Could you check a few things on this model? Use its own coordinates, in mm. Face numbers are marked on the shaded views. Give positions to 0.01 mm unless a question says otherwise; leave off trailing zeros. Loops run counter-clockwise (first coordinate to the right, second up) from the corner with the lowest first, then second, coordinate; pieces in that order, holes last. Notation, with made-up numbers: (-10.75, 80.25) - (42.25, 80.25) arc R30 cw to (42.25, 113.25) - close; hole circle Ø9 at (-9, -6.75). An arc over 180 degrees is marked (long way). Write each question's results on one line, items separated by ' | '. Start each with the question number.
(1) I need wall thicknesses on line 1 (Y direction, x = -1, z = 2.6); line 2 (X direction, y = 4.5, z = 2.7); line 3 (X direction, y = -0.5, z = 0.8) (3 decimals). Which ranges of each line are inside material? Lowest first, please.
(2) Suppose I cut it at A-A (y = 5.5). Please give me the cut outline in (x, z), and give its area (3 significant figures).
(3) Suppose I cut it at B-B (y = 1.5). Please give me the cut outline in (x, z), and give its area (3 significant figures).
(4) For pin 1 (4 mm diameter, centred on x = 0, y = 0, fed in from +Z); pin 2 (1.5 mm diameter, centred on x = -6.5, z = 1.5, fed in from +Y), each with a flat end and sliding along its axis, tell me the tip position at first contact or that it passes through.
(5) Suppose I cut it at C-C (x = 0). Please give me the cut outline in (y, z).
(6) Suppose I cut it at D-D (y = -7.5). Please give me the cut outline in (x, z), and give its area (3 significant figures).
(7) If we mould it in two halves opening along Y, with no side actions, what happens to the marked faces 1, 2, 3 and 4? For each: released by +Y, released by -Y, zero draft, split by the parting line, or undercut.
from build123d import *

# Parameters (mm, degrees)
SKETCH_1_R      = 3
SKETCH_1_R_2    = 0.8
SKETCH_1_R_3    = 1.25
EXTRUDE_1_DEPTH = 3
FILLET_1_R      = 0.5
FILLET_2_R      = 1


with BuildPart() as part:
    # ｽｹｯﾁ1 → ﾎﾞｽ - 押し出し1 (new body)
    with BuildSketch(Plane.XY):
        with BuildLine():
            ThreePointArc((-11.50012809, -9.630527187), (-15.242047107, -8.8), (-14.090345241, -5.144139479))
            ThreePointArc((-14.090345241, -5.144139479), (-12.990381057, 7.5), (-2.590217151, 14.774666667))
            ThreePointArc((-2.590217151, 14.774666667), (0, 17.6), (2.590217151, 14.774666667))
            ThreePointArc((2.590217151, 14.774666667), (12.990381057, 7.5), (14.090345241, -5.144139479))
            ThreePointArc((14.090345241, -5.144139479), (15.242047107, -8.8), (11.50012809, -9.630527187))
            ThreePointArc((11.50012809, -9.630527187), (0, -15), (-11.50012809, -9.630527187))
        make_face()
        with Locations((-8.749968889, 2.106666667)):
            Circle(SKETCH_1_R, mode=Mode.SUBTRACT)
        with Locations((0, -6.75)):
            Circle(SKETCH_1_R, mode=Mode.SUBTRACT)
        with Locations((0, 15)):
            Circle(SKETCH_1_R_2, mode=Mode.SUBTRACT)
        with Locations((12.990381057, -7.5)):
            Circle(SKETCH_1_R_2, mode=Mode.SUBTRACT)
        with Locations((-12.990381057, -7.5)):
            Circle(SKETCH_1_R_2, mode=Mode.SUBTRACT)
        with Locations((-7.109225892, -3.668638333)):
            Circle(SKETCH_1_R_3, mode=Mode.SUBTRACT)
        with Locations((7.109225892, 3.668638333)):
            Circle(SKETCH_1_R_3, mode=Mode.SUBTRACT)
        with BuildLine():
            ThreePointArc((1.563335837, 2.849294836), (0.895749756, 8.670249526), (-0.94779451, 3.108727323))
            ThreePointArc((-0.94779451, 3.108727323), (-0.333989648, -3.232793052), (1.563335837, 2.849294836))
        make_face(mode=Mode.SUBTRACT)
    extrude(amount=EXTRUDE_1_DEPTH)

    # ﾌｨﾚｯﾄ1
    fillet_1_edges = [part.edges().sort_by_distance(p)[0] for p in [
        (-0.94779451, 3.108727323, 1.5),
        (1.563335837, 2.849294836, 1.5),
    ]]
    fillet(fillet_1_edges, radius=FILLET_1_R)

    # ﾌｨﾚｯﾄ2
    fillet_2_edges = [part.edges().sort_by_distance(p)[0] for p in [
        (-11.50012809, -9.630527187, 1.5),
        (-14.090345241, -5.144139479, 1.5),
        (-2.590217151, 14.774666667, 1.5),
        (2.590217151, 14.774666667, 1.5),
        (14.090345241, -5.144139479, 1.5),
        (11.50012809, -9.630527187, 1.5),
    ]]
    fillet(fillet_2_edges, radius=FILLET_2_R)


solid = part.part
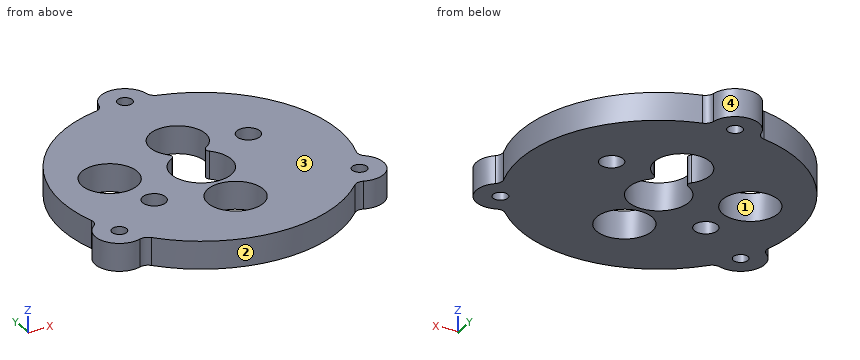
Output values:
1) line 1: -14.97 to -9.58, -3.92 to -3.09, 8.23 to 17.4 | line 2: -14.31 to -10.56, -6.94 to -2.17, 3.34 to 6.18, 8.04 to 14.31 | line 3: -14.992 to -10.235, -7.265 to -3.211, 3.211 to 14.992
2) outline: (-13.96, 0) - (-2.41, 0) - (-2.41, 3) - (-13.96, 3) - close; (3.58, 0) - (13.96, 0) - (13.96, 3) - (3.58, 3) - close | area: 65.8 mm2
3) outline: (-14.92, 0) - (-11.69, 0) - (-11.69, 3) - (-14.92, 3) - close; (-5.81, 0) - (-2.88, 0) - (-2.88, 3) - (-5.81, 3) - close; (2.88, 0) - (14.92, 0) - (14.92, 3) - (2.88, 3) - close | area: 54.6 mm2
4) pin 1: through | pin 2: y = 13.85
5) outline: (-15, 0) - (-9.75, 0) - (-9.75, 3) - (-15, 3) - close; (-3.75, 0) - (-3.25, 0) - (-3.25, 3) - (-3.75, 3) - close; (8.63, 0) - (14.2, 0) - (14.2, 3) - (8.63, 3) - close; (15.8, 0) - (17.6, 0) - (17.6, 3) - (15.8, 3) - close
6) outline: (-15.59, 0) - (-13.79, 0) - (-13.79, 3) - (-15.59, 3) - close; (-12.19, 0) - (-2.9, 0) - (-2.9, 3) - (-12.19, 3) - close; (2.9, 0) - (12.19, 0) - (12.19, 3) - (2.9, 3) - close; (13.79, 0) - (15.59, 0) - (15.59, 3) - (13.79, 3) - close | area: 66.5 mm2
7) face 1: undercut | face 2: released by -Y | face 3: zero draft | face 4: released by +Y
